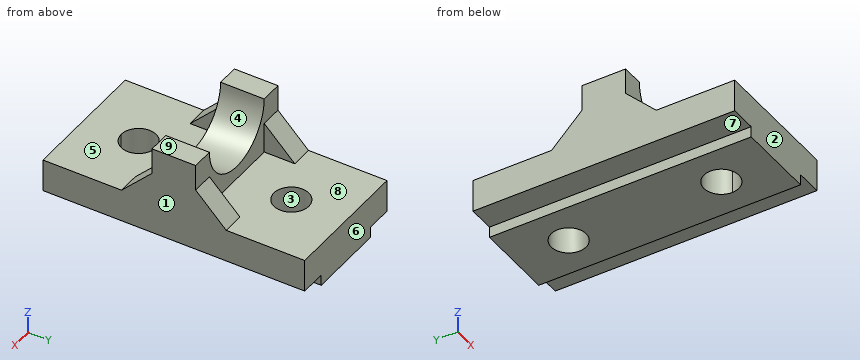
```python
from build123d import *

# Parameters (mm, degrees)
F0_W          = 60
F0_H          = 120
F1_DEPTH      = 20
F2_W          = 12
F2_H          = 5
F3_DEPTH      = 258.3
F5_DEPTH      = 30
F5_DEPTH_BACK = 30
F6_R          = 20
F7_DEPTH      = 64
F7_DEPTH_BACK = 66
F8_R          = 8
F9_DEPTH      = 44.3
F11_DEPTH     = 115
F12_W         = 40
F12_H         = 14
F13_DEPTH     = 57
F14_DEPTH     = 49


with BuildPart() as f1:
    # F0 (on Top) → F1 (new body)
    with BuildSketch(Plane.XY):
        Rectangle(F0_W, F0_H)
    extrude(amount=F1_DEPTH)

    # F2 (on face) → F3 (cut)
    with BuildSketch(Plane.XZ.offset(60)):
        with Locations((-24, 2.5)):
            Rectangle(F2_W, F2_H)
        with Locations((24, 2.5)):
            Rectangle(F2_W, F2_H)
    extrude(amount=-F3_DEPTH, mode=Mode.SUBTRACT)

    # F4 (on Right) → F5 (join, two sides)
    with BuildSketch(Plane.YZ) as f5_sk:
        Polygon((0, 46), (0, 20), (24, 20), (10, 34), (10, 46), align=None)
        Polygon((-24, 20), (0, 20), (0, 46), (-10, 46), (-10, 34), align=None)
    extrude(amount=F5_DEPTH)
    extrude(f5_sk.sketch, amount=-F5_DEPTH_BACK)

    # F6 (on face) → F7 (cut, two sides)
    with BuildSketch(Plane(origin=(0, 10, 0), x_dir=(-1, 0, 0), z_dir=(0, 1, 0))) as f7_sk:
        with Locations((0, 46)):
            Circle(F6_R)
    extrude(amount=-F7_DEPTH, mode=Mode.SUBTRACT)
    extrude(f7_sk.sketch, amount=F7_DEPTH_BACK, mode=Mode.SUBTRACT)

    # F8 (on face) → F9 (cut)
    with BuildSketch(Plane.XY.offset(20)):
        with BuildLine():
            ThreePointArc((0, -43), (5.6568542495, -40.6568542495), (8, -35))
            ThreePointArc((8, -35), (-5.6568542495, -29.3431457505), (0, -43))
        make_face()
        with Locations((0, 35)):
            Circle(F8_R)
    extrude(amount=-F9_DEPTH, mode=Mode.SUBTRACT)

    # F10 (on Top) → F11 (cut)
    with BuildSketch(Plane.XY):
        Polygon((20, -10), (-16, -10), (-20, -10), (-20, -24), (16, -24), (20, -24), align=None)
    extrude(amount=F11_DEPTH, mode=Mode.SUBTRACT)

    # F12 (on Top) → F13 (cut)
    with BuildSketch(Plane.XY):
        with Locations((0, 17)):
            Rectangle(F12_W, F12_H)
    extrude(amount=F13_DEPTH, mode=Mode.SUBTRACT)

    # F14 (add): a face of the model
    f14_faces = [f1.faces().sort_by_distance(p)[0] for p in [
        (0, 24, 10.1923076923),
    ]]
    extrude(f14_faces, amount=F14_DEPTH)


solid = f1.part
```
Geometry check sheet. Reference: the model listing, model coordinates, mm. Face numbers are marked on the shaded views. A direction names the side the tool comes from. Coordinates: 2 decimals unless noted, no trailing zeros. Write each loop counter-clockwise with the first axis right and the second up, starting at its lowest first coordinate (ties: lowest second). Pieces come first, ordered by that corner, then holes. Notation, with made-up numbers: (74, 82.5) -> (94, 82.5) arc R14 ccw to (94, 101.5) -> close; hole circle Ø7 at (-29, 41.5). An arc over 180 degrees is marked (long way). Use CSV: the item, a comma, the result in double quotes. Start each with the question number.
Item 1: Mould release check, pull along X, two halves, no side actions. Record for the marked faces 1, 2, 3 and 4: released by +X, released by -X, zero draft, split by the parting line, or undercut.
Item 2: Cross-section at C-C, the plane x = 22.5. Record the cut outline in (y, z), plus the area to 3 significant figures.
Item 3: Thickness scan on line 1 (Y direction, x = 0, z = 8); line 2 (X direction, y = 11, z = 26); line 3 (Z direction, x = 8.5, y = -12.5). Record the ranges inside material, lowest first.
Item 4: Set-up check for the marked faces 5, 6, 7, 8 and 9: record each of +Z, -Z, +X, -X, +Y, -Y from which the full face is reachable in a straight line by a thin tool's end or side.
Item 5: Cross-section at D-D, the plane y = 52. Record the cut outline in (x, z), plus the area to 3 significant figures.
Item 6: Cross-section at B-B, the plane y = -30. Record the cut outline in (x, z) (3 decimals), plus the area to 3 significant figures.
Item 7: Depth check by flat-ended pin: pin 1 Ø8 at (x, z) = (3, 30.5) entering from -Y; pin 2 Ø25 at (x, y) = (-3.5, 30) entering from +Z; pin 3 Ø4 at (y, z) = (-30, 2) entering from +X; pin 4 Ø3.5 at (x, y) = (-25.5, -10) entering from -Z. Enter the tip coordinate at first touch or a pass-through.
Item 8: Cross-section at A-A, the plane z = 15.5. Record the cut outline in (x, y), plus the area to 3 significant figures.
Answers:
1,face 1,"released by +X"
1,face 2,"zero draft"
1,face 3,"undercut"
1,face 4,"undercut"
2,outline,"(-60, 5) -> (60, 5) -> (60, 20) -> (24, 20) -> (10, 34) -> (10, 46) -> (-10, 46) -> (-10, 34) -> (-24, 20) -> (-60, 20) -> close"
2,area,"2,520 mm^2"
3,line 1,"-60 to -43, -27 to 27, 43 to 60"
3,line 2,"-30 to -20, 20 to 30"
3,line 3,"0 to 20"
4,face 5,"+Z, -Y"
4,face 6,"+Z, -Z, +X, -X, +Y"
4,face 7,"-Z, -X, +Y, -Y"
4,face 8,"+Z, +Y"
4,face 9,"+Z, +X, -X, +Y, -Y"
5,outline,"(-30, 5) -> (-18, 5) -> (-18, 0) -> (18, 0) -> (18, 5) -> (30, 5) -> (30, 20) -> (-30, 20) -> close"
5,area,"1,080 mm^2"
6,outline,"(-30, 5) -> (-18, 5) -> (-18, 0) -> (-6.245, 0) -> (-6.245, 20) -> (-30, 20) -> close; (6.245, 0) -> (18, 0) -> (18, 5) -> (30, 5) -> (30, 20) -> (6.245, 20) -> close"
6,area,"830 mm^2"
7,pin 1,"through"
7,pin 2,"z = 20"
7,pin 3,"x = 18"
7,pin 4,"z = 5"
8,outline,"(-30, -60) -> (30, -60) -> (30, 60) -> (-30, 60) -> close; hole circle Ø16 at (0, -35); hole circle Ø16 at (0, 35)"
8,area,"6,800 mm^2"
